from build123d import *

# Parameters (mm, degrees)
SKETCH_1_W          = 28.5
SKETCH_1_H          = 20
SKETCH_1_R          = 2.5
EXTRUDE_1_DEPTH     = 4.5
CHAMFER_1_SIZE      = 2.5
SKETCH_2_R          = 15
CUT_EXTRUDE_1_DEPTH = 5.5


with BuildPart() as part:
    # Эскиз1 → Бобышка-Вытянуть1 (new body)
    with BuildSketch(Plane.XY):
        Rectangle(SKETCH_1_W, SKETCH_1_H)
        with Locations((9.25, 5)):
            Circle(SKETCH_1_R, mode=Mode.SUBTRACT)
    extrude(amount=EXTRUDE_1_DEPTH)

    # Фаска1
    chamfer_1_edges = [part.edges().sort_by_distance(p)[0] for p in [
        (14.25, 10, 2.25),
    ]]
    chamfer(chamfer_1_edges, length=CHAMFER_1_SIZE)

    # Зеркальное отражение1: part across plane


with BuildPart() as part_1:
    add(part.part)
    add(part.part.mirror(Plane(origin=(-14.25, -10, 4.5), x_dir=(0, 0, 1), z_dir=(0, 1, 0))))

    # Зеркальное отражение2: part across plane


with BuildPart() as part_2:
    add(part_1.part)
    add(part_1.part.mirror(Plane(origin=(-14.25, -10, 4.5), x_dir=(0, 0, 1), z_dir=(1, 0, 0))))

    # Эскиз2 → Вырез-Вытянуть1 (cut, through all)
    with BuildSketch(Plane.XY.offset(4.5)):
        with Locations((-14.25, -10)):
            Circle(SKETCH_2_R)
    extrude(amount=-CUT_EXTRUDE_1_DEPTH, mode=Mode.SUBTRACT)


solid = part_2.part
Could you check a few things on this model? Use its own coordinates, in mm. Give positions to 0.01 mm unless a question says otherwise; leave off trailing zeros. Order: outer loops, then holes, each group sorted by start corner. A loop starts at its lowest first (then second) coordinate and runs counter-clockwise, first axis right, second up. Notation, with made-up numbers: (88.25, 50) - (114.25, 50) arc R23 ccw to (114.25, 87) - close; hole circle Ø11 at (20.5, 30.5). An arc over 180 degrees is marked (long way). Return JSON: item names as keys, results as strings. Group by question number.
Q1. Will these pins go through, and if not, where does the flat tip stop? pin 1 Ø6.5 at (x, y) = (9.25, -25) entering from +Z; pin 2 Ø1 at (x, y) = (-27.5, -8) entering from -Z.
Q2. Suppose I cut it at C-C, the plane x = -15. Please give me the cut outline in (y, z), and give its area (3 significant figures).
Q3. Thinking about a two-plate mould opening in Y: for faces 1 (the face through (-14, 10, 2)), 2 (the face through (8.92, -27.48, 2.22)), 3 (the face through (-8, -24, 4.5)), which applies, pulls with the +Y half, pulls with the -Y half, needs draft (parallel to the pull), parting line crosses it, or undercut?
Q4. Suppose I cut it at B-B, the plane x = -37.75. Please give me the cut outline in (y, z), and give its area (3 significant figures).
Q5. Please list where these lines run through material, in increasing order: line 1 along Y through (x, z) = (9.25, 1.8); line 2 along Y through (x, z) = (-37, 2.8); line 3 along X through (y, z) = (-9.5, 1.25). Write a range as [from, to].
Q6. Suppose I cut it at A-A, the plane y = -10. Please give me the cut outline in (x, z), and give its area (4 significant figures).
Resolved:
{
 "1": {"pin 1": "stops at z = 4.5", "pin 2": "passes through"},
 "2": {"outline": "(-30, 0) - (-24.98, 0) - (-24.98, 4.5) - (-30, 4.5) - close; (4.98, 0) - (10, 0) - (10, 4.5) - (4.98, 4.5) - close", "area": "45.2 mm2"},
 "3": {"face 1": "pulls with the +Y half", "face 2": "undercut", "face 3": "needs draft"},
 "4": {"outline": "(-30, 0) - (-27.5, 0) - (-27.5, 4.5) - (-30, 4.5) - close; (-22.5, 0) - (2.5, 0) - (2.5, 4.5) - (-22.5, 4.5) - close; (7.5, 0) - (10, 0) - (10, 4.5) - (7.5, 4.5) - close", "area": "135 mm2"},
 "5": {"line 1": "y = [-30, -27.5], [-22.5, 2.5], [7.5, 10]", "line 2": "y = [-30, -27.38], [-22.62, 2.62], [7.38, 10]", "line 3": "x = [-42.75, -29.24], [0.74, 14.25]"},
 "6": {"outline": "(-42.75, 0) - (-29.25, 0) - (-29.25, 4.5) - (-42.75, 4.5) - close; (0.75, 0) - (14.25, 0) - (14.25, 4.5) - (0.75, 4.5) - close", "area": "121.5 mm2"}
}
